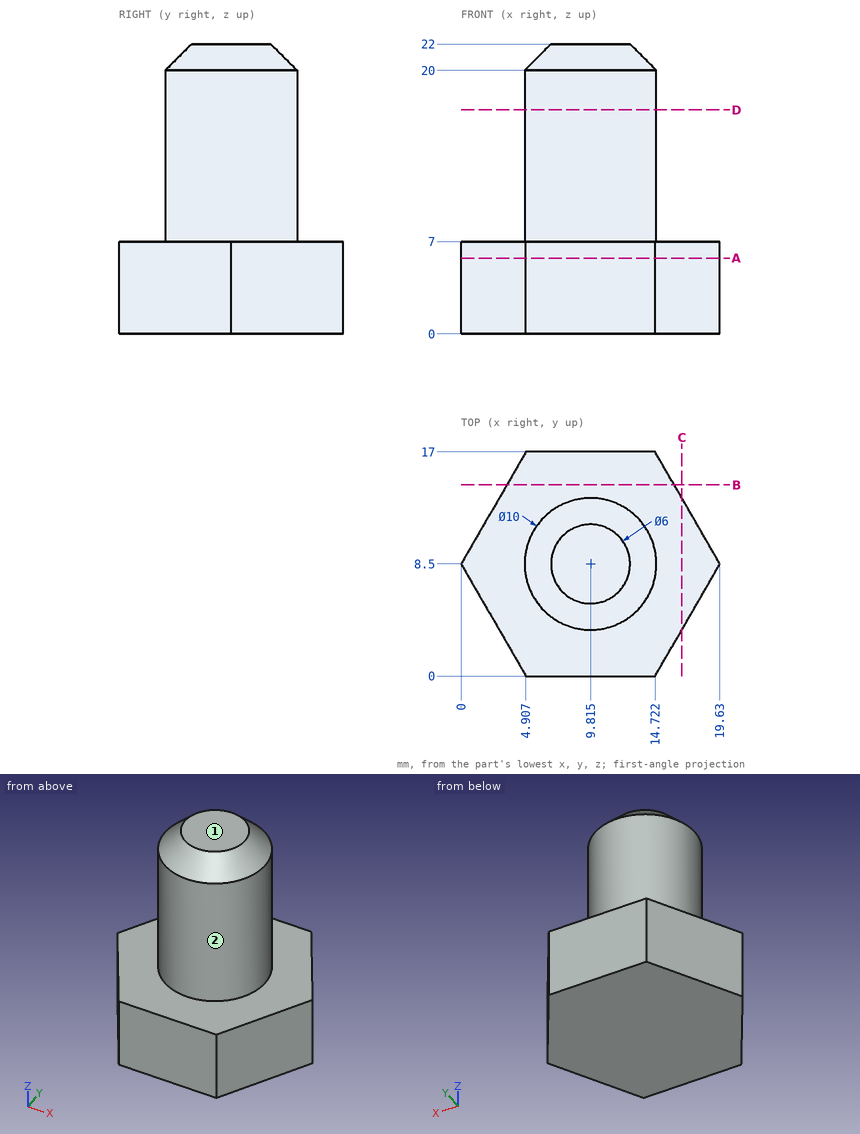
The figure shows three views and two pictorial views of one solid part (mm, origin at its lowest corner). Answer the questions. A direction names the side the tool comes from. Give positions to 0.01 mm unless a question says otherwise; leave off trailing zeros. Order: outer loops, then holes, each group sorted by start corner. A loop starts at its lowest first (then second) coordinate and runs counter-clockwise, first axis right, second up. Notation, with made-up numbers: (89, 5) -> (114, 5) arc R11 cw to (114, 14) -> close; hole circle Ø8 at (65.25, 5.5). An arc over 180 degrees is marked (long way). Answer as a JSON object with one key per item and string values. Group by question number.
Item 1: The part is cut by section D-D on z = 17. Write down the section's boundary in (x, y) (1 decimal).
Item 2: The part is cut by section B-B on y = 14.5. Write down the section's boundary in (x, z) (1 decimal), and give its area (3 significant figures).
Item 3: A tool of negligible diameter and unlimited length cuts with its end or side. For the marked faces 1 and 2, from which of +Z, -Z, +X, -X, +Y, -Y can it reach the whole face along a straight path? Write none if from no direction.
Item 4: The part is cut by section C-C on x = 16.75. Write down the section's boundary in (y, z).
Item 5: Consider L1, parallel to Z at x = 15.25, y = 6.75; L2, parallel to Y at x = 18.5, z = 4.5 (1 decimal); L3, parallel to X at y = 6.75, z = 17.75. Determine where each line is inside the solid, lowest interval first. Write a range as from..to.
Item 6: The part is cut by section A-A on z = 5.75. Write down the section's boundary in (x, y), and give its area (3 significant figures).
Item 7: Flat-ended cylindrical pins translate along their axes: pin 1 (1 mm diameter, centred on y = 10, z = 13.5, fed in from -X); pin 2 (1 mm diameter, centred on x = 12.5, z = 14, fed in from +Y); pin 3 (2 mm diameter, centred on x = 2, z = 5.5, fed in from +Y) (1 decimal). Find the tip coordinate at first contact, or state that the pin passes through.
Result set:
{
 "1": {"outline": "circle Ø10 at (9.8, 8.5)"},
 "2": {"outline": "(3.5, 0) -> (16.2, 0) -> (16.2, 7) -> (3.5, 7) -> close", "area": "88.9 mm²"},
 "3": {"face 1": "+Z, +X, -X, +Y, -Y", "face 2": "+Z"},
 "4": {"outline": "(3.51, 0) -> (13.49, 0) -> (13.49, 7) -> (3.51, 7) -> close"},
 "5": {"L1": "0..7", "L2": "6.5..10.5", "L3": "5.13..14.5"},
 "6": {"outline": "(0, 8.5) -> (4.91, 0) -> (14.72, 0) -> (19.63, 8.5) -> (14.72, 17) -> (4.91, 17) -> close", "area": "250 mm²"},
 "7": {"pin 1": "x = 4.92", "pin 2": "y = 13", "pin 3": "y = 13.7"}
}
